from build123d import *

# Parameters (mm, degrees)
F0_W     = 110
F0_H     = 80
F1_DEPTH = 7
F2_W     = 100.000002
F2_H     = 70.000002
F3_DEPTH = 3.5
F4_R     = 5
F5_R     = 10
F6_R     = 1.5


with BuildPart() as f1:
    # F0 (on Top) → F1 (new body)
    with BuildSketch(Plane.XY):
        Rectangle(F0_W, F0_H)
    extrude(amount=F1_DEPTH)

    # F2 (on face) → F3 (cut)
    with BuildSketch(Plane.XY.offset(7)):
        Rectangle(F2_W, F2_H)
    extrude(amount=-F3_DEPTH, mode=Mode.SUBTRACT)

    # F4
    f4_edges = [f1.edges().sort_by_distance(p)[0] for p in [
        (50.000001, -35.000001, 5.25),
        (-50.000001, -35.000001, 5.25),
        (-50.000001, 35.000001, 5.25),
        (50.000001, 35.000001, 5.25),
    ]]
    fillet(f4_edges, radius=F4_R)

    # F5
    f5_edges = [f1.edges().sort_by_distance(p)[0] for p in [
        (-55, -40, 3.5),
        (55, -40, 3.5),
        (55, 40, 3.5),
        (-55, 40, 3.5),
    ]]
    fillet(f5_edges, radius=F5_R)

    # F6
    f6_edges = [f1.edges().sort_by_distance(p)[0] for p in [
        (0, -40, 7),
        (50.000001, 0, 7),
    ]]
    fillet(f6_edges, radius=F6_R)


solid = f1.part
Here's how the part is built. I have some questions about the finished solid (model axes, mm). A direction names the side the tool comes from. Round coordinates to 2 decimals unless told otherwise and drop trailing zeros. Write each loop counter-clockwise with the first axis right and the second up, starting at its lowest first coordinate (ties: lowest second). Pieces come first, ordered by that corner, then holes. Notation, with made-up numbers: (-10, -37.5) -> (45, -37.5) arc R13 ccw to (45, -28.5) -> close; hole circle Ø9 at (-2.75, 39). An arc over 180 degrees is marked (long way). One line per item, written item: value.
1) If I drill on line 1 (Y direction, x = 40, z = 3.75); line 2 (X direction, y = 11, z = 5); line 3 (Z direction, x = -4, y = -23.5), over which ranges is the centre line in solid material (lowest first)? Write a range as [from, to].
Filled sheet:
line 1: y = [-40, -35], [35, 40]
line 2: x = [-55, -50], [50, 55]
line 3: z = [0, 3.5]
2) For faces 4 (the face through (-52.15, 36.99, 2.79)), 5 (the face through (48, -34, 4)), which set-ups out of +Z, -Z, +X, -X, +Y, -Y let a thin tool reach every point of the face, with its end or its side?
Filled sheet:
face 4: +Z, -Z, -X, +Y
face 5: +Z
3) Suppose I cut it at A-A on y = -15. List the corners of the cut face in (x, z) for me.
Filled sheet:
outline: (-55, 0) -> (55, 0) -> (55, 5.5) arc R1.5 ccw to (53.5, 7) -> (51.5, 7) arc R1.5 ccw to (50, 5.5) -> (50, 3.5) -> (-50, 3.5) -> (-50, 5.5) arc R1.5 ccw to (-51.5, 7) -> (-53.5, 7) arc R1.5 ccw to (-55, 5.5) -> close
4) I'm going to push flat-ended pins straight in: pin 1 Ø3 at (y, z) = (5.5, 6) entering from -X; pin 2 Ø10 at (x, y) = (-15.5, 21.5) entering from +Z. Where does each tip first touch, or does it pass through?
Filled sheet:
pin 1: stops at x = -55
pin 2: stops at z = 3.5
5) Suppose I cut it at B-B on x = -3.5. List the corners of the cut face in (y, z) for me.
Filled sheet:
outline: (-40, 0) -> (40, 0) -> (40, 5.5) arc R1.5 ccw to (38.5, 7) -> (36.5, 7) arc R1.5 ccw to (35, 5.5) -> (35, 3.5) -> (-35, 3.5) -> (-35, 5.5) arc R1.5 ccw to (-36.5, 7) -> (-38.5, 7) arc R1.5 ccw to (-40, 5.5) -> close
6) We'd pull the mould along X, two halves only. Please class faces 1 (the face through (-55, 0, 3)), 2 (the face through (-52, 0, 7)), 3 (the face through (-48, 34, 4)): released by +X, released by -X, zero draft, split by the parting line, or undercut.
Filled sheet:
face 1: released by -X
face 2: zero draft
face 3: undercut
